Verification items for the finished model (mm, model axes). A direction names the side the tool comes from. Coordinates: 2 decimals unless noted, no trailing zeros. Loops run counter-clockwise (first coordinate to the right, second up) from the corner with the lowest first, then second, coordinate; pieces in that order, holes last. Notation, with made-up numbers: (46, -39) - (101, -39) arc R15 cw to (101, -19) - close; hole circle Ø6 at (5.5, 34.25). An arc over 180 degrees is marked (long way). One line per item, written item: value. Start each with the question number.
(1) Set-up check for faces 1 (the face through (7.5, 2, 16)), 2 (the face through (-6, 3, 16)), 3 (the face through (-20, 3, -3)): record each of +Z, -Z, +X, -X, +Y, -Y from which the full face is reachable in a straight line by a thin tool's end or side.
(2) Section check D-D (z = 6.5). Record the boundary of the cut face in (x, y).
(3) Section check C-C (x = 25.5). Record the boundary of the cut face in (y, z).
(4) Section check B-B (y = 3.35). Record the boundary of the cut face in (x, z), plus the area to 3 significant figures.
(5) Section check A-A (z = 21.5). Record the boundary of the cut face in (x, y), plus the area to 3 significant figures.
(6) Draft check along Z on faces 4 (the face through (12.274, 2.535, 10.698)), 5 (the face through (20, 3, -3)), 6 (the face through (0, 0, 10)). Enter one of: +Z half, -Z half, draft (parallel to the pull), parting line (faces both ways), or undercut.
(7) Thickness scan on probe 1 along X at (y, z) = (2.9, 2.5); probe 2 along X at (y, z) = (3.55, 14); probe 3 along Z at (x, y) = (2, 4). Record the ranges inside material, lowest first. Write a range as [from, to].
(8) Gauge pin test, flat ends, axial feed: P1, Ø2.5, axis at x = -23, y = 1.5, coming from the -Z side; P2, Ø3, axis at x = -9, y = 1, coming from the -Z side; P3, Ø7.5, axis at x = 0, z = 0, coming from the +Y side; P4, Ø2.5, axis at y = 3.5, z = 19.5, coming from the +X side. Record the tip position at first contact, or that the pin passes through.
```python
from build123d import *

# Parameters (mm, degrees)
SKETCH1_R           = 4.1
SKETCH1_R_2         = 6.3
BOSS_EXTRUDE1_DEPTH = 5
FILLET1_R           = 3
CUT_EXTRUDE1_DEPTH  = 43.720018727
SKETCH3_R           = 6
CUT_EXTRUDE2_DEPTH  = 43.60278036


with BuildPart() as part:
    # Sketch1 → Boss-Extrude1 (new body)
    # profile 1 of 2: a face of its own
    with BuildSketch(Plane(origin=(0, 0, 0), x_dir=(1, 0, 0), z_dir=(0, 1, 0))):
        with BuildLine():
            Line((0, -30), (0, -12.5))
            ThreePointArc((0, -12.5), (3.75, -8.75), (7.5, -12.5))
            Line((7.5, -12.5), (7.5, -19.267848855))
            ThreePointArc((7.5, -19.267848855), (13.800000007, -12.967848868), (20.1, -19.267848868))
            ThreePointArc((20.1, -19.267848868), (19.403598453, -22.147030066), (17.468354167, -24.3896823))
            ThreePointArc((17.468354167, -24.3896823), (26.683802437, -13.710386117), (30, 0))
            ThreePointArc((30, 0), (-21.213203436, 21.213203436), (0, -30))
        make_face()
        with Locations(Location((0, 0, 0), (0, 0, 270))):
            Circle(SKETCH1_R, mode=Mode.SUBTRACT)
    # profile 2 of 2: a face of its own
    with BuildSketch(Plane(origin=(0, 0, 0), x_dir=(1, 0, 0), z_dir=(0, 1, 0))):
        with Locations((13.8, -19.267848868)):
            Circle(SKETCH1_R_2)
    extrude(amount=BOSS_EXTRUDE1_DEPTH)

    # Fillet1
    fillet1_edges = [part.edges().sort_by_distance(p)[0] for p in [
        (0, 2.5, 30),
    ]]
    fillet(fillet1_edges, radius=FILLET1_R)

    # Sketch2 → Cut-Extrude1 (cut, through all)
    with BuildSketch(Plane(origin=(0, 5, 0), x_dir=(1, 0, 0), z_dir=(0, 1, 0))):
        with BuildLine():
            Line((-24, 3), (-23.8117618, 3))
            ThreePointArc((-23.8117618, 3), (0, 24), (23.8117618, 3))
            Line((23.8117618, 3), (24, 3))
            Line((24, 3), (29.849623113, 3))
            ThreePointArc((29.849623113, 3), (0, 30), (-29.849623113, 3))
            Line((-29.849623113, 3), (-24, 3))
        make_face()
        with BuildLine():
            ThreePointArc((23.8117618, 3), (0, 24), (-23.8117618, 3))
            Line((-23.8117618, 3), (-9.644169223, 3))
            ThreePointArc((-9.644169223, 3), (0, 10.1), (9.644169223, 3))
            Line((9.644169223, 3), (23.8117618, 3))
        make_face()
        with BuildLine():
            ThreePointArc((-23.8117618, -3), (-18.016060482, -15.856278401), (-6, -23.237900077))
            Line((-6, -23.237900077), (-6, -8.124653839))
            ThreePointArc((-6, -8.124653839), (-8.231070824, -5.85315924), (-9.644169223, -3))
            Line((-9.644169223, -3), (-23.8117618, -3))
        make_face()
    extrude(amount=-CUT_EXTRUDE1_DEPTH, mode=Mode.SUBTRACT)

    # Sketch3 → Cut-Extrude2 (cut, through all)
    with BuildSketch(Plane(origin=(0, 5, 0), x_dir=(1, 0, 0), z_dir=(0, 1, 0))):
        with Locations(Location((17.596672685, -7.929343091, 0), (0, 0, 270))):
            Circle(SKETCH3_R)
    extrude(amount=-CUT_EXTRUDE2_DEPTH, mode=Mode.SUBTRACT)


solid = part.part
```
Responses:
1. face 1: +Z, +Y, -Y
1. face 2: +Y, -Y
1. face 3: -Z, -X, +Y, -Y
2. outline: (-29.29, 0) - (-23.1, 0) - (-23.1, 5) - (-29.29, 5) - close; (-7.73, 0) - (11.77, 0) - (11.77, 5) - (-7.73, 5) - close; (23.42, 0) - (29.29, 0) - (29.29, 5) - (23.42, 5) - close
3. outline: (0, -3) - (5, -3) - (5, 15.8) - (0, 15.8) - close
4. outline: (-29.85, -3) - (-9.64, -3) arc R10.1 ccw to (9.64, -3) - (29.85, -3) arc R30 ccw to (17.47, 24.39) arc R6.3 ccw to (7.5, 19.27) - (7.5, 12.5) arc R3.75 cw to (0, 12.5) - (0, 26.83) arc R3 ccw to (-3.33, 29.81) arc R30 ccw to start; hole (-23.81, 3) - (-9.64, 3) arc R10.1 cw to (-6, 8.12) - (-6, 23.24) arc R24 ccw to start; hole circle Ø8.2 at (0, 0); hole circle Ø12 at (17.6, 7.93)
4. area: 1,110 mm²
5. outline: (-20.92, 0) - (-10.67, 0) - (-10.67, 5) - (-20.92, 5) - close; (-6, 0) - (0, 0) - (0, 5) - (-6, 5) - close; (7.91, 0) - (20.92, 0) - (20.92, 5) - (7.91, 5) - close
5. area: 146 mm²
6. face 4: undercut
6. face 5: -Z half
6. face 6: draft
7. probe 1: x = [-29.9, -3.25], [3.25, 15.04], [20.15, 29.9]
7. probe 2: x = [-26.53, -19.49], [-6, 0], [7.5, 26.53]
7. probe 3: z = [-9.9, -3.58], [3.58, 9.18]
8. P1: stops at z = -3
8. P2: stops at z = -6.76
8. P3: passes through
8. P4: stops at x = 23.81
